Check sheet for the modelled part. Datum: model origin and axes. Units: mm. A direction names the side the tool comes from. Give positions to 0.01 mm unless a question says otherwise; leave off trailing zeros. Order: outer loops, then holes, each group sorted by start corner. A loop starts at its lowest first (then second) coordinate and runs counter-clockwise, first axis right, second up.
Item 1: Sectioned sample at C-C on z = 23.5. Record the boundary of the cut face in (x, y), and give its area (3 significant figures).
Item 2: Material ranges on line 1 along X through (y, z) = (-1.25, 47); line 2 along X through (y, z) = (-1.25, 46); line 3 along Z through (x, y) = (-7, -1.75), recorded low to high.
Item 3: Access from +Z, -Z, +X, -X, +Y, -Y to the whole of each face (thin tool, end or side, straight path). Record for faces 4 (the cylindrical face through (-27.231, -0.496, -49.256)), 5 (the cylindrical face through (12.476, -0.632, 52.395)).
Item 4: Gauge pin test, flat ends, axial feed: P1, Ø1, axis at y = 2.5, z = -3, coming from the -X side; P2, Ø2, axis at x = -14, y = 0, coming from the +Z side. Record the tip position at first contact, or that the pin passes through.
Item 5: Sectioned sample at B-B on z = 47. Record the boundary of the cut face in (x, y), and give its area (3 significant figures).
Item 6: Sectioned sample at A-A on x = 0. Record the boundary of the cut face in (y, z), and give its area (3 significant figures).
Item 7: Sectioned sample at D-D on z = -38. Record the boundary of the cut face in (x, y).
Item 8: Release check for a two-part mould opening along X. For faces 1 (the cylindrical face through (-40.482, -0.056, -25.186)), 2 (the flat face through (-41.61, 0.06, -43.24)), 3 (the flat face through (0, 0, 60)) record: released by +X, released by -X, zero draft, split by the parting line, or undercut.
from build123d import *

# Parameters (mm, degrees)
SKETCH_2_R                  = 40
EXTRUDE_1_DEPTH             = 4
HOLE_WIZARD_M3_1_D          = 3.4
HOLE_WIZARD_M4_1_AT_2_COUNT = 2
HOLE_WIZARD_M4_1_AT_2_PITCH = 28
HOLE_WIZARD_M4_3_D          = 3.3
HOLE_WIZARD_M4_3_DEPTH      = 15
HOLE_WIZARD_M4_3_TIP        = 0.991420021
HOLE_WIZARD_M4_1_2_D        = 4.3


with BuildPart() as part:
    # 草图2 → 凸台-拉伸1 (new, symmetric)
    with BuildSketch(Plane(origin=(0, 0, 0), x_dir=(1, 0, 0), z_dir=(0, 1, 0))):
        Polygon((20, 64.852813742), (-20, 64.852813742), (-63.840620434, 21.012193309), (-35, -60), (35, -60), (63.840620434, 21.012193309), align=None)
        with Locations(Location((0, 0, 0), (0, 0, 270))):
            Circle(SKETCH_2_R, mode=Mode.SUBTRACT)
    extrude(amount=EXTRUDE_1_DEPTH, both=True)

    # M3 间隙孔1 (through all)
    with Locations(Plane(origin=(0, 4, 0), x_dir=(1, 0, 0), z_dir=(0, 1, 0))):
        with Locations((0, 47), (40.703193978, 23.5), (40.703193978, -23.5), (0, -47), (-40.703193978, -23.5), (-40.703193978, 23.5)):
            Hole(HOLE_WIZARD_M3_1_D / 2)

    # 草图7 → Hole Wizard M4 _1 (revolve, cut)
    with BuildSketch(Plane(origin=(32.526911935, 0, -52.325901808), x_dir=(-0.7071067811865476, 0, -0.7071067811865476), z_dir=(0, 1, 0))):
        Polygon((0, 0), (0, 12.991420021), (1.65, 12), (1.65, 0), align=None)
    hole_wizard_m4_1 = revolve(axis=Axis((37.017039995, 0, -56.816029868), (-0.7071067811865476, 0, 0.7071067811865476)), mode=Mode.SUBTRACT)

    # Hole Wizard M4 _1 at 2: Hole Wizard M4 _1 ×2
    with Locations(*[Vector(0.7071067811865476, 0, 0.7071067811865476) * (i * HOLE_WIZARD_M4_1_AT_2_PITCH) for i in range(1, HOLE_WIZARD_M4_1_AT_2_COUNT)]):
        add(hole_wizard_m4_1, mode=Mode.SUBTRACT)

    # 镜向1: Hole Wizard M4 _1 across plane
    add(hole_wizard_m4_1.mirror(Plane(origin=(0, 0, 0), x_dir=(0, 0, 1), z_dir=(1, 0, 0))), mode=Mode.SUBTRACT)

    # 镜向1 copy 1 sketch → 镜向1 copy 1 (revolve, cut)
    with BuildSketch(Plane(origin=(-52.325901808, 0, -32.526911935), x_dir=(0.7071067811865476, 0, -0.7071067811865476), z_dir=(0, 1, 0))):
        Polygon((0, 0), (0, -12.991420021), (1.65, -12), (1.65, 0), align=None)
    revolve(axis=Axis((-56.816029868, 0, -37.017039995), (-0.7071067811865476, 0, -0.7071067811865476)), mode=Mode.SUBTRACT)

    # M4 螺纹孔3
    with Locations(Plane.XY.offset(60)):
        with Locations((14, 0), (-14, 0)):
            Hole(HOLE_WIZARD_M4_3_D / 2, depth=HOLE_WIZARD_M4_3_DEPTH)
            with Locations((0, 0, -(HOLE_WIZARD_M4_3_DEPTH + HOLE_WIZARD_M4_3_TIP / 2))):  # 118° drill point
                Cone(0, HOLE_WIZARD_M4_3_D / 2, HOLE_WIZARD_M4_3_TIP, mode=Mode.SUBTRACT)

    # Hole Wizard M4 _1 2 (through all)
    with Locations(Plane(origin=(0, 4, 0), x_dir=(1, 0, 0), z_dir=(0, 1, 0))):
        with Locations((-7, 57.852813742), (7, 57.852813742)):
            Hole(HOLE_WIZARD_M4_1_2_D / 2)


solid = part.part
Report:
1. outline: (-47.99, -4) - (-42.4, -4) - (-42.4, 4) - (-47.99, 4) - close; (-39, -4) - (-32.37, -4) - (-32.37, 4) - (-39, 4) - close; (32.37, -4) - (39, -4) - (39, 4) - (32.37, 4) - close; (42.4, -4) - (47.99, -4) - (47.99, 4) - (42.4, 4) - close
1. area: 196 mm2
2. line 1: x = -39.63 to -15.08, -12.92 to -1.7, 1.7 to 12.92, 15.08 to 39.63
2. line 2: x = -39.98 to -15.08, -12.92 to -1.37, 1.37 to 12.92, 15.08 to 39.98
2. line 3: z = -64.85 to -60, -55.7 to -39.38, 39.38 to 60
3. face 4: none
3. face 5: +Z
4. P1: stops at x = -57.61
4. P2: stops at z = 44.61
5. outline: (-39.63, -4) - (-1.7, -4) - (-1.7, 4) - (-39.63, 4) - close; (1.7, -4) - (39.63, -4) - (39.63, 4) - (1.7, 4) - close; hole circle Ø3.3 at (-14, 0); hole circle Ø3.3 at (14, 0)
5. area: 590 mm2
6. outline: (-4, -64.85) - (4, -64.85) - (4, -48.7) - (-4, -48.7) - close; (-4, -45.3) - (4, -45.3) - (4, -40) - (-4, -40) - close; (-4, 40) - (4, 40) - (4, 45.3) - (-4, 45.3) - close; (-4, 48.7) - (4, 48.7) - (4, 60) - (-4, 60) - close
6. area: 304 mm2
7. outline: (-46.85, -4) - (-12.49, -4) - (-12.49, 4) - (-46.85, 4) - close; (12.49, -4) - (46.85, -4) - (46.85, 4) - (12.49, 4) - close
8. face 1: undercut
8. face 2: released by -X
8. face 3: zero draft
